from build123d import *

# Parameters (mm, degrees)
SKETCH1_R           = 3.175
SKETCH1_R_2         = 1.27
BOSS_EXTRUDE1_DEPTH = 3.175


with BuildPart() as part:
    # Sketch1 → Boss-Extrude1 (new body)
    with BuildSketch(Plane.XY):
        with BuildLine():
            Line((115.57, 0), (128.27, 0))
            Line((128.27, 0), (134.683820715, -6.413820715))
            Line((134.683820715, -6.413820715), (116.017803308, -25.079838122))
            Line((116.017803308, -25.079838122), (146.157549282, -11.59220999))
            ThreePointArc((146.157549282, -11.59220999), (153.389965114, 2.652256881), (140.97, 12.7))
            Line((140.97, 12.7), (0, 12.7))
            ThreePointArc((0, 12.7), (-12.7, 0), (0, -12.7))
            Line((0, -12.7), (115.442358569, -12.7))
            Line((115.442358569, -12.7), (109.156179285, -6.413820715))
            Line((109.156179285, -6.413820715), (115.57, 0))
        make_face()
        Circle(SKETCH1_R, mode=Mode.SUBTRACT)
        with Locations((140.97, 0)):
            Circle(SKETCH1_R_2, mode=Mode.SUBTRACT)
    extrude(amount=BOSS_EXTRUDE1_DEPTH)


solid = part.part
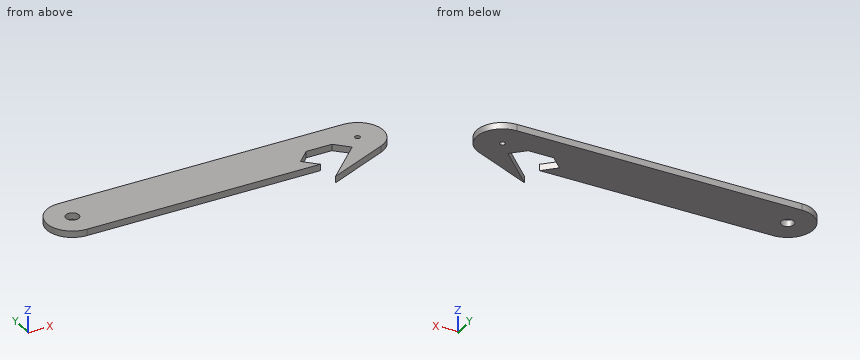
Check sheet for the modelled part. Datum: model origin and axes. Units: mm. Give positions to 0.01 mm unless a question says otherwise; leave off trailing zeros. Write each loop counter-clockwise with the first axis right and the second up, starting at its lowest first coordinate (ties: lowest second). Pieces come first, ordered by that corner, then holes. Notation, with made-up numbers: M 89.5,-38.75 L 132.5,-38.75 A26 ccw 132.5,-12.75 Z; hole C 10.5,80 d10. An arc over 180 degrees is marked long. Use one line per item in the form item = value.
(1) Section check C-C on x = 19. Record the boundary of the cut face in (y, z) (3 decimals).
Answer block:
outline = M -12.7,0 L 12.7,0 L 12.7,3.175 L -12.7,3.175 Z
(2) Section check A-A on z = 0.8. Record the boundary of the cut face in (x, y) (3 decimals), plus the area to 3 significant figures.
Answer block:
outline = M 0,-12.7 L 115.442,-12.7 L 109.156,-6.414 L 115.57,0 L 128.27,0 L 134.684,-6.414 L 116.018,-25.08 L 146.158,-11.592 A12.7 ccw 140.97,12.7 L 0,12.7 A12.7 ccw Z; hole C 0,0 d6.35; hole C 140.97,0 d2.54
area = 3,900 mm2
(3) Depth check by flat-ended pin: P1, Ø1.5, axis at y = -18, z = 2.5, coming from the +X side; P2, Ø1, axis at x = 49.5, z = 1.5, coming from the -Y side; P3, Ø1.6, axis at x = 121.5, z = 2, coming from the -Y side. Enter the tip coordinate at first touch or a pass-through.
Answer block:
P1 = 133.51
P2 = -12.7
P3 = -22.98
(4) Material ranges on line 1 along Y through (x, z) = (0, 2.4) (3 decimals); line 2 along Y through (x, z) = (33, 2.7); line 3 along X through (y, z) = (2, 2.9), recorded low to high.
Answer block:
line_1 = -12.7 to -3.175, 3.175 to 12.7
line_2 = -12.7 to 12.7
line_3 = -12.54 to -2.47, 2.47 to 153.51
(5) Section check B-B on y = -9.5. Record the boundary of the cut face in (x, z) (3 decimals), plus the area to 3 significant figures.
Answer block:
outline = M -8.429,0 L 112.242,0 L 112.242,3.175 L -8.429,3.175 Z; M 131.598,0 L 149.399,0 L 149.399,3.175 L 131.598,3.175 Z
area = 440 mm2
